Verification items for the finished model (mm, model axes). Round coordinates to 2 decimals unless told otherwise and drop trailing zeros. Order: outer loops, then holes, each group sorted by start corner. A loop starts at its lowest first (then second) coordinate and runs counter-clockwise, first axis right, second up. Notation, with made-up numbers: M 86,62 L 115,62 A20 ccw 115,97 Z; hole C 33,73.5 d2. An arc over 180 degrees is marked long. One line per item, written item: value. Start each with the question number.
from build123d import *

# Parameters (mm, degrees)
ESQUISSE1_W      = 80
ESQUISSE1_H      = 100
EXTRUSION1_DEPTH = 6
ESQUISSE2_R      = 8
EXTRUSION3_DEPTH = 129.202964084
ESQUISSE3_R      = 3
EXTRUSION4_DEPTH = 129.202964084
EXTRUSION5_DEPTH = 129.202964084
CHANFREIN1_SIZE  = 2


with BuildPart() as part:
    # Esquisse1 → Extrusion1 (new body)
    with BuildSketch(Plane(origin=(0, 0, 0), x_dir=(0, 0, -1), z_dir=(1, 0, 0))):
        with Locations((40, 50)):
            Rectangle(ESQUISSE1_W, ESQUISSE1_H)
    extrude(amount=EXTRUSION1_DEPTH)

    # Esquisse2 → Extrusion3 (cut, through all)
    with BuildSketch(Plane(origin=(6, 0, 0), x_dir=(0, 0, -1), z_dir=(1, 0, 0))):
        with Locations((40, 77)):
            Circle(ESQUISSE2_R)
        with Locations((40, 30)):
            Circle(ESQUISSE2_R)
    extrude(amount=-EXTRUSION3_DEPTH, mode=Mode.SUBTRACT)

    # Esquisse3 → Extrusion4 (cut, through all)
    with BuildSketch(Plane(origin=(6, 0, 0), x_dir=(0, 0, -1), z_dir=(1, 0, 0))):
        with Locations((10, 95)):
            Circle(ESQUISSE3_R)
        with Locations(Location((70, 95, 0), (0, 0, 180))):
            Circle(ESQUISSE3_R)
        with Locations((20, 5)):
            Circle(ESQUISSE3_R)
        with Locations(Location((60, 5, 0), (0, 0, 180))):
            Circle(ESQUISSE3_R)
    extrude(amount=-EXTRUSION4_DEPTH, mode=Mode.SUBTRACT)

    # Esquisse4 → Extrusion5 (cut, through all)
    with BuildSketch(Plane(origin=(6, 0, 0), x_dir=(0, 0, -1), z_dir=(1, 0, 0))):
        with BuildLine():
            Line((14.5, 88), (23.568323275, 88))
            ThreePointArc((23.568323275, 88), (25.703928765, 86.799688112), (25.78882013, 84.351351351))
            ThreePointArc((25.78882013, 84.351351351), (24.18182416, 74.59473222), (28.616262416, 65.756756757))
            ThreePointArc((28.616262416, 65.756756757), (29.144270989, 63.036125499), (26.837553419, 61.5))
            Line((26.837553419, 61.5), (14.5, 61.5))
            ThreePointArc((14.5, 61.5), (12.732233047, 62.232233047), (12, 64))
            Line((12, 64), (12, 85.5))
            ThreePointArc((12, 85.5), (12.732233047, 87.267766953), (14.5, 88))
        make_face()
        with BuildLine():
            Line((12, 56.5), (40, 56.5))
            ThreePointArc((40, 56.5), (43, 53.5), (40, 50.5))
            Line((40, 50.5), (12, 50.5))
            ThreePointArc((12, 50.5), (9, 53.5), (12, 56.5))
        make_face()
        with BuildLine():
            Line((14.5, 45.5), (26.837553419, 45.5))
            ThreePointArc((26.837553419, 45.5), (29.144270989, 43.963874501), (28.616262416, 41.243243243))
            ThreePointArc((28.616262416, 41.243243243), (24.029537881, 29.028228573), (30.063459206, 17.459459459))
            ThreePointArc((30.063459206, 17.459459459), (30.871875411, 14.678005063), (28.510874707, 13))
            Line((28.510874707, 13), (14.5, 13))
            ThreePointArc((14.5, 13), (12.732233047, 13.732233047), (12, 15.5))
            Line((12, 15.5), (12, 43))
            ThreePointArc((12, 43), (12.732233047, 44.767766953), (14.5, 45.5))
        make_face()
        with BuildLine():
            Line((65.5, 13), (51.489125293, 13))
            ThreePointArc((51.489125293, 13), (49.128124589, 14.678005063), (49.936540794, 17.459459459))
            ThreePointArc((49.936540794, 17.459459459), (55.974264455, 30.907124639), (48.452969685, 43.584818861))
            ThreePointArc((48.452969685, 43.584818861), (47.310016798, 45.28313862), (47.818996959, 47.265957447))
            ThreePointArc((47.818996959, 47.265957447), (50, 53.5), (47.818996959, 59.734042553))
            ThreePointArc((47.818996959, 59.734042553), (47.310016798, 61.71686138), (48.452969685, 63.415181139))
            ThreePointArc((48.452969685, 63.415181139), (55.427142463, 72.756973317), (54.21117987, 84.351351351))
            ThreePointArc((54.21117987, 84.351351351), (54.296071235, 86.799688112), (56.431676725, 88))
            Line((56.431676725, 88), (65.5, 88))
            ThreePointArc((65.5, 88), (67.267766953, 87.267766953), (68, 85.5))
            Line((68, 85.5), (68, 15.5))
            ThreePointArc((68, 15.5), (67.267766953, 13.732233047), (65.5, 13))
        make_face()
    extrude(amount=-EXTRUSION5_DEPTH, mode=Mode.SUBTRACT)

    # Chanfrein1
    chanfrein1_edges = [part.edges().sort_by_distance(p)[0] for p in [
        (6, 95, -7),
        (6, 95, -73),
        (6, 5, -17),
        (6, 5, -63),
    ]]
    chamfer(chanfrein1_edges, length=CHANFREIN1_SIZE - 0.0001)  # a hair under: the kernel refuses the full size


solid = part.part
1. Section check D-D (y = 30). Record the cut outline in (x, z), and give its area (3 significant figures).
2. Draft check along Y on faces 1 (the face through (0, 51, -48)), 2 (the face through (3, 13, -22)). Enter one of: released by +Y, released by -Y, zero draft, split by the parting line, or undercut.
3. Section check A-A (z = -20). Give the number of separate pieces and of enclosed holes in the cut face, and give its area (3 significant figures).
4. Depth check by flat-ended pin: pin 1 (8 mm diameter, centred on y = 62.5, z = -62.5, fed in from -X). Enter the tip coordinate at first touch or a pass-through.
5. Section check B-B (y = 53.5). Record the cut outline in (x, z), and give its area (3 significant figures).
6. Scan lines: line 1 along Y through (x, z) = (1.75, -40); line 2 along Y through (x, z) = (2, -60); line 3 along Y through (x, z) = (1.1, -20). Record each from-to range of solid material in increasing order.
Geometry check:
1. outline: M 0,-80 L 6,-80 L 6,-68 L 0,-68 Z; M 0,-56 L 6,-56 L 6,-48 L 0,-48 Z; M 0,-32 L 6,-32 L 6,-24 L 0,-24 Z; M 0,-12 L 6,-12 L 6,0 L 0,0 Z
1. area: 240 mm²
2. face 1: zero draft
2. face 2: undercut
3. separate pieces: 5
3. enclosed holes: 0
3. area: 170 mm²
4. pin 1: passes through
5. outline: M 0,-80 L 6,-80 L 6,-68 L 0,-68 Z; M 0,-50 L 6,-50 L 6,-43 L 0,-43 Z; M 0,-9 L 6,-9 L 6,0 L 0,0 Z
5. area: 168 mm²
6. line 1: y = 0 to 22, 38 to 50.5, 56.5 to 69, 85 to 100
6. line 2: y = 0 to 2, 8 to 13, 88 to 100
6. line 3: y = 0 to 2, 8 to 13, 45.5 to 50.5, 56.5 to 61.5, 88 to 100
